Print and shaded views of the part. All mm, measured from the part's lowest x, y and z. Coordinates: 2 decimals unless noted, no trailing zeros. Order: outer loops, then holes, each group sorted by start corner. A loop starts at its lowest first (then second) coordinate and runs counter-clockwise, first axis right, second up. Notation, with made-up numbers: (51.25, -15.5) - (87.25, -15.5) arc R37 cw to (87.25, 22.5) - close; hole circle Ø8 at (-36.75, 9.25). An arc over 180 degrees is marked (long way). Write each question's results on one line, items separated by ' | '.
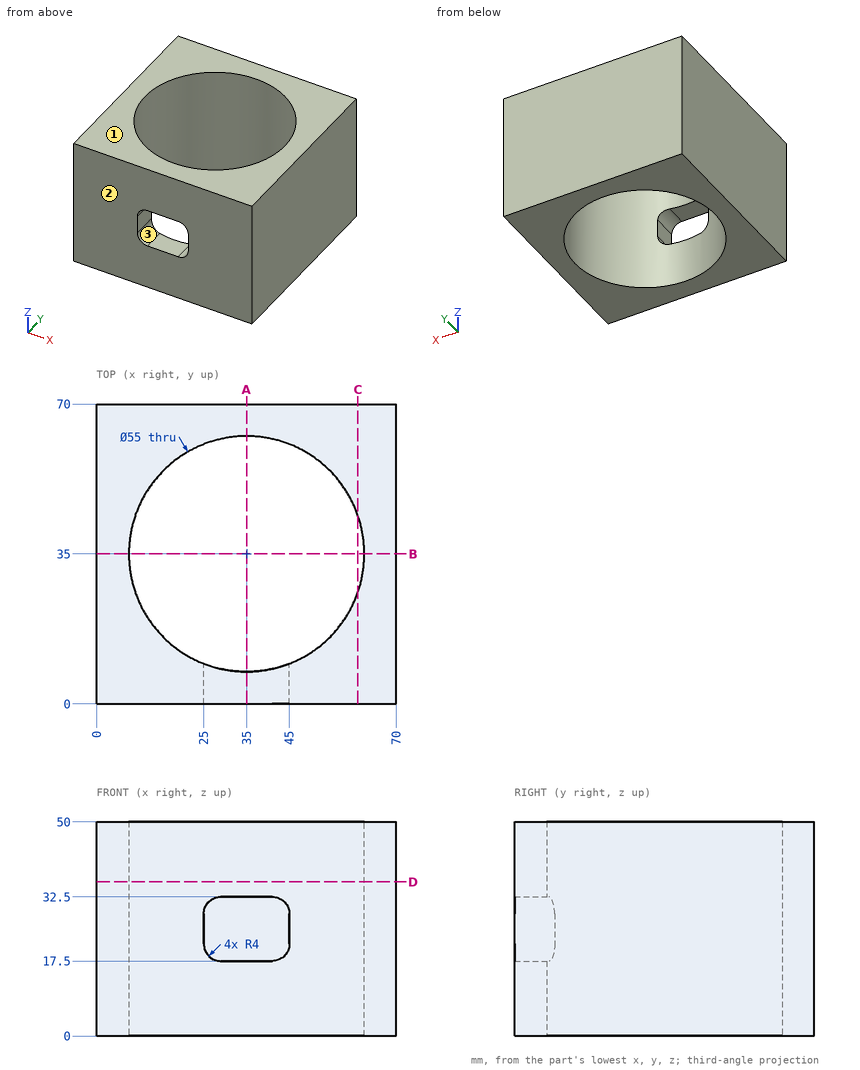
1. Band-saw the part on D-D on z = 36. Give the cut face in (x, y), then the cut area to 3 significant figures.
Solved:
outline: (0, 0) - (70, 0) - (70, 70) - (0, 70) - close; hole circle Ø55 at (35, 35) | area: 2,520 mm2
2. Band-saw the part on B-B on y = 35. Give the cut face in (x, z).
Solved:
outline: (0, 0) - (7.5, 0) - (7.5, 50) - (0, 50) - close; (62.5, 0) - (70, 0) - (70, 50) - (62.5, 50) - close
3. Band-saw the part on C-C on x = 61. Give the cut face in (y, z).
Solved:
outline: (0, 0) - (26.04, 0) - (26.04, 50) - (0, 50) - close; (43.96, 0) - (70, 0) - (70, 50) - (43.96, 50) - close
4. Band-saw the part on A-A on x = 35. Give the cut face in (y, z), then the cut area to 4 significant figures.
Solved:
outline: (0, 0) - (7.5, 0) - (7.5, 17.5) - (0, 17.5) - close; (0, 32.5) - (7.5, 32.5) - (7.5, 50) - (0, 50) - close; (62.5, 0) - (70, 0) - (70, 50) - (62.5, 50) - close | area: 637.5 mm2
5. Probe line 1 (Y direction, x = 35, z = 39); line 2 (Y direction, x = 35, z = 22); line 3 (Y direction, x = 20.5, z = 9). List the from-to ranges inside material, lowest first.
Solved:
line 1: y = 0 to 7.5, 62.5 to 70 | line 2: y = 62.5 to 70 | line 3: y = 0 to 11.63, 58.37 to 70
6. Two-plate mould, pull along Z, no slides. Class the marked faces 1, 2 and 3: +Z half, -Z half, draft (parallel to the pull), parting line (faces both ways), or undercut.
Solved:
face 1: +Z half | face 2: draft | face 3: undercut
